```python
from build123d import *

# Parameters (mm, degrees)
F1_DEPTH = 19
F2_R     = 20
F3_DEPTH = 10
F5_DEPTH = 3
F6_R     = 4
F7_DEPTH = 7


with BuildPart() as f1:
    # F0 (on Front) → F1 (new body, symmetric)
    with BuildSketch(Plane.XZ):
        with BuildLine():
            ThreePointArc((-15, 0), (0, 15), (15, 0))
            Line((15, 0), (50, 0))
            Line((50, 0), (50, 7))
            Line((50, 7), (24, 7))
            ThreePointArc((24, 7), (0, 25), (-24, 7))
            Line((-24, 7), (-50, 7))
            Line((-50, 7), (-50, 0))
            Line((-50, 0), (-15, 0))
        make_face()
    extrude(amount=F1_DEPTH, both=True)

    # F2 (on Front) → F3 (cut, symmetric)
    with BuildSketch(Plane.XZ):
        Circle(F2_R)
    extrude(amount=F3_DEPTH, both=True, mode=Mode.SUBTRACT)

    # F4 (on Front) → F5 (join, symmetric)
    with BuildSketch(Plane.XZ):
        with BuildLine():
            Line((-30, 25), (-30, 7))
            Line((-30, 7), (-24, 7))
            ThreePointArc((-24, 7), (0, 25), (24, 7))
            Line((24, 7), (30, 7))
            Line((30, 7), (30, 25))
            ThreePointArc((30, 25), (28.535534, 28.535534), (25, 30))
            Line((25, 30), (-25, 30))
            ThreePointArc((-25, 30), (-28.535534, 28.535534), (-30, 25))
        make_face()
    extrude(amount=F5_DEPTH, both=True)

    # F6 (on face) → F7 (cut, through all)
    with BuildSketch(Plane.XY.offset(7)):
        with Locations((-40, -11)):
            Circle(F6_R)
        with Locations((40, -11)):
            Circle(F6_R)
        with Locations((-40, 0)):
            Circle(F6_R)
        with Locations((40, 0)):
            Circle(F6_R)
        with Locations((-40, 11)):
            Circle(F6_R)
        with Locations((40, 11)):
            Circle(F6_R)
    extrude(amount=-F7_DEPTH, mode=Mode.SUBTRACT)


solid = f1.part
```
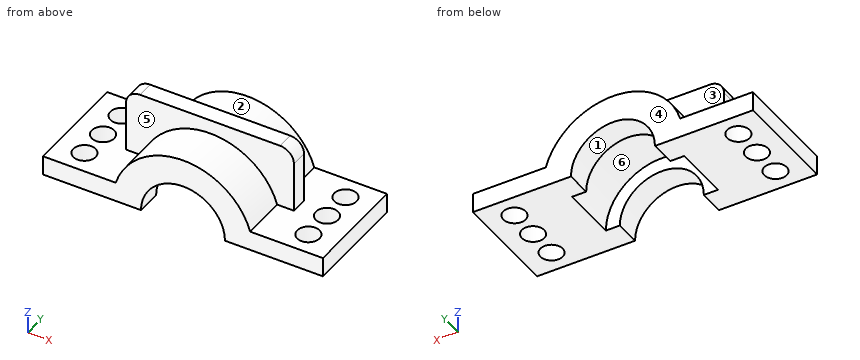
Source: CAD feature listing. Evaluate the final solid. Frame: model axes, mm. Face numbers are marked on the shaded views. A direction names the side the tool comes from. Give positions to 0.01 mm unless a question says otherwise; leave off trailing zeros. Write each loop counter-clockwise with the first axis right and the second up, starting at its lowest first coordinate (ties: lowest second). Pieces come first, ordered by that corner, then holes.
1. Section query D-D (z = 17.5). Return the cut outline in (x, y).
2. Access query for the marked faces 4, 5 and 6. Directions: +Z, -Z, +X, -X, +Y, -Y. A direction counts if a zero-diameter tool reaches every point of the face in a straight line with its end or side. Return the directions, or none.
3. Section query B-B (x = 40). Return the cut outline in (y, z).
4. Section query A-A (y = 0). Return the cut outline in (x, z).
5. Material intervals for line 1 along Y through (x, z) = (-40, 1.5); line 2 along Z through (x, y) = (-44.5, -8); line 3 along X through (y, z) = (-13, 7.5), sorted ascending.
6. Pull-direction query (X, two-part tool) for the marked faces 1, 2 and 3; classes: +X half, -X half, draft (parallel to the pull), parting line (faces both ways), or undercut.
7. First-contact query: pin 1 (5 mm diameter, centred on x = 40, y = -11, fed in from -Z); pin 2 (9 mm diameter, centred on x = 40, y = 0, fed in from +Z); pin 3 (6.5 mm diameter, centred on y = -1.5, z = 18, fed in from -X); pin 4 (8 mm diameter, centred on y = -12.5, z = 24.5, fed in from -X). Flat tips, straight axial feed; report the tip coordinate or a pass-through.
8. Section query C-C (x = 0). Return the cut outline in (y, z), then the cut area to 3 significant figures.
Output values:
1. outline: (-30, -3) - (-17.85, -3) - (-17.85, -19) - (17.85, -19) - (17.85, -3) - (30, -3) - (30, 3) - (17.85, 3) - (17.85, 19) - (-17.85, 19) - (-17.85, 3) - (-30, 3) - close; hole (-9.68, -10) - (9.68, -10) - (9.68, 10) - (-9.68, 10) - close
2. face 4: +Z, -Z, +X, -X, +Y
2. face 5: +Z, -Y
2. face 6: -Z
3. outline: (-19, 0) - (-15, 0) - (-15, 7) - (-19, 7) - close; (-7, 0) - (-4, 0) - (-4, 7) - (-7, 7) - close; (4, 0) - (7, 0) - (7, 7) - (4, 7) - close; (15, 0) - (19, 0) - (19, 7) - (15, 7) - close
4. outline: (-50, 0) - (-44, 0) - (-44, 7) - (-50, 7) - close; (-36, 0) - (-20, 0) arc R20 cw to (20, 0) - (36, 0) - (36, 7) - (30, 7) - (30, 25) arc R5 ccw to (25, 30) - (-25, 30) arc R5 ccw to (-30, 25) - (-30, 7) - (-36, 7) - close; (44, 0) - (50, 0) - (50, 7) - (44, 7) - close
5. line 1: y = -19 to -15, -7 to -4, 4 to 7, 15 to 19
5. line 2: z = 0 to 7
5. line 3: x = -23.85 to -12.99, 12.99 to 23.85
6. face 1: undercut
6. face 2: parting line
6. face 3: draft
7. pin 1: passes through
7. pin 2: stops at z = 7
7. pin 3: stops at x = -30
7. pin 4: stops at x = -14.31
8. outline: (-19, 15) - (-10, 15) - (-10, 20) - (10, 20) - (10, 15) - (19, 15) - (19, 25) - (3, 25) - (3, 30) - (-3, 30) - (-3, 25) - (-19, 25) - close
8. area: 310 mm2
